For this review, take the finished solid that the model builds, in its own axes (mm). A direction names the side the tool comes from. Round coordinates to 2 decimals unless told otherwise and drop trailing zeros. Write each loop counter-clockwise with the first axis right and the second up, starting at its lowest first coordinate (ties: lowest second). Pieces come first, ordered by that corner, then holes. Notation, with made-up numbers: (63, 7) -> (120, 7) arc R11 cw to (120, 15) -> close; hole circle Ø6 at (14, 33). An arc over 180 degrees is marked (long way). Answer as CSV lines item,"result". Start each with the question number.
Item 1: For pin 1 Ø1.2 at (x, y) = (0.5, 1) entering from -Z; pin 2 Ø1.5 at (x, y) = (-2.5, -1) entering from +Z; pin 3 Ø1.5 at (y, z) = (0.5, 1) entering from +X, all flat-tipped, find the tip position at first contact; note any pin that passes through.
Item 2: Take a section at C-C on y = 0.9. Give the boundary of the cut face in (x, z).
Item 3: Wall thickness on probe 1 along Y at (x, z) = (3.25, -2); probe 2 along X at (y, z) = (0.5, 1.25); probe 3 along Z at (x, y) = (-1.75, -0.8): over which ranges is each line inside the solid? List them lowest first. Write a range as from..to.
Item 4: Take a section at A-A on z = 0. Give the boundary of the cut face in (x, y).
Item 5: Take a section at D-D on y = -0.3. Give the boundary of the cut face in (x, z).
Item 6: Take a section at B-B on x = 0. Give the boundary of the cut face in (y, z).
Item 7: Machinability: for faces 1 (the flat face through (-2.5, 1, 0)), 2 (the flat face through (2.5, 1, 0)), 3 (the flat face through (0, 1, -2.5)), which of the approach directions +Z, -Z, +X, -X, +Y, -Y give a long, thin tool a straight path to every point of the face, cutting with its end or side? Answer none if there is none.
```python
from build123d import *

# Parameters (mm, degrees)
SKETCH1_R           = 4.75
BOSS_EXTRUDE1_DEPTH = 1.2
SKETCH2_W           = 5
SKETCH2_H           = 5
BOSS_EXTRUDE2_DEPTH = 1.5


with BuildPart() as part:
    # Sketch1 → Boss-Extrude1 (new body)
    with BuildSketch(Plane(origin=(0, 0, 0), x_dir=(1, 0, 0), z_dir=(0, 1, 0))):
        with Locations(Location((0, 0, 0), (0, 0, 270))):
            Circle(SKETCH1_R)
    extrude(amount=-BOSS_EXTRUDE1_DEPTH)

    # Sketch2 → Boss-Extrude2 (add)
    with BuildSketch(Plane(origin=(0, 0, 0), x_dir=(1, 0, 0), z_dir=(0, 1, 0))):
        Rectangle(SKETCH2_W, SKETCH2_H)
    extrude(amount=BOSS_EXTRUDE2_DEPTH)


solid = part.part
```
Output values:
1,pin 1,"stops at z = -2.5"
1,pin 2,"stops at z = 4.42"
1,pin 3,"stops at x = 4.73"
2,outline,"(-2.5, -2.5) -> (2.5, -2.5) -> (2.5, 2.5) -> (-2.5, 2.5) -> close"
3,probe 1,"y = -1.2..0"
3,probe 2,"x = -2.5..2.5"
3,probe 3,"z = -4.42..4.42"
4,outline,"(-4.75, -1.2) -> (4.75, -1.2) -> (4.75, 0) -> (2.5, 0) -> (2.5, 1.5) -> (-2.5, 1.5) -> (-2.5, 0) -> (-4.75, 0) -> close"
5,outline,"circle Ø9.5 at (0, 0)"
6,outline,"(-1.2, -4.75) -> (0, -4.75) -> (0, -2.5) -> (1.5, -2.5) -> (1.5, 2.5) -> (0, 2.5) -> (0, 4.75) -> (-1.2, 4.75) -> close"
7,face 1,"+Z, -Z, -X, +Y"
7,face 2,"+Z, -Z, +X, +Y"
7,face 3,"-Z, +X, -X, +Y"
